from build123d import *

# Parameters (mm, degrees)
F0_W     = 25.4
F0_H     = 19.05
F0_R     = 5.08
F1_DEPTH = 2.032
F3_DEPTH = 19.05


with BuildPart() as f1:
    # F0 (on Top) → F1 (new body)
    with BuildSketch(Plane.XY):
        Rectangle(F0_W, F0_H)
        with Locations((-2.54, 0)):
            Circle(F0_R, mode=Mode.SUBTRACT)
    extrude(amount=F1_DEPTH)

    # F2 (on face) → F3 (join, through all)
    with BuildSketch(Plane.XZ.offset(9.525)):
        Polygon((10.16, 2.032), (12.7, 2.032), (12.7, 7.112), (3.482183, 7.112), (3.482183, 2.032), (4.752183, 2.032), (4.752183, 4.572), (10.16, 4.572), align=None)
    extrude(amount=-F3_DEPTH)


solid = f1.part
Design review of the part built by this model. Coordinates are the model's own, in mm. A direction names the side the tool comes from. Round coordinates to 2 decimals unless told otherwise and drop trailing zeros. Loops run counter-clockwise (first coordinate to the right, second up) from the corner with the lowest first, then second, coordinate; pieces in that order, holes last. Notation, with made-up numbers: (46.5, 30) -> (94.5, 30) arc R32 cw to (94.5, 61) -> close; hole circle Ø7 at (78, 53). An arc over 180 degrees is marked (long way). Use one line per item in the form item = value. Start each with the question number.
Q1. Draft analysis for pull direction Z (two halves, no side actions). For faces 1 (the face through (12.7, 0, 4)), 2 (the face through (8, 0, 7.112)), 3 (the face through (10.16, 0, 3)), 4 (the face through (3, 0, 0)), state which applies: +Z half, -Z half, draft (parallel to the pull), parting line (faces both ways), or undercut.
Q2. We need section B-B on x = 7.25. Give the boundary of the cut face in (y, z) (3 decimals).
Q3. We need section A-A on y = 0. Give the boundary of the cut face in (x, z).
Q4. Wall thickness on line 1 along X through (y, z) = (-0.25, 4); line 2 along Z through (x, y) = (6.25, 0.5); line 3 along Y through (x, z) = (-2.54, 1.05) (3 decimals): over which ranges is each line inside the solid? List them lowest first. Write a range as [from, to].
Q5. For pin 1 Ø8 at (x, y) = (-2, -2) entering from +Z; pin 2 Ø4 at (x, z) = (1, 5) entering from +Y; pin 3 Ø1.5 at (y, z) = (4, 3.5) entering from -X, all flat-tipped, find the tip position at first contact; note any pin that passes through.
Q6. We need section D-D on y = -7. Give the boundary of the cut face in (x, z), then the cut area to 3 significant figures.
Q7. We need section C-C on z = 3.5. Give the boundary of the cut face in (x, y) (3 decimals), then the cut area to 3 significant figures.
Q8. Machinability: for faces 5 (the face through (4.752, 0, 3)), 6 (the face through (-8, 0, 2.032)), 7 (the face through (2.305, 1.526, 1.002)), which of the approach directions +Z, -Z, +X, -X, +Y, -Y give a long, thin tool a straight path to every point of the face, cutting with its end or side? Answer none if there is none.
Calculated:
q1.face_1 = draft
q1.face_2 = +Z half
q1.face_3 = undercut
q1.face_4 = -Z half
q2.outline = (-9.525, 0) -> (9.525, 0) -> (9.525, 2.032) -> (-9.525, 2.032) -> close; (-9.525, 4.572) -> (9.525, 4.572) -> (9.525, 7.112) -> (-9.525, 7.112) -> close
q3.outline = (-12.7, 0) -> (-7.62, 0) -> (-7.62, 2.03) -> (-12.7, 2.03) -> close; (2.54, 0) -> (12.7, 0) -> (12.7, 7.11) -> (3.48, 7.11) -> (3.48, 2.03) -> (2.54, 2.03) -> close; hole (4.75, 2.03) -> (10.16, 2.03) -> (10.16, 4.57) -> (4.75, 4.57) -> close
q4.line_1 = [3.48, 4.75], [10.16, 12.7]
q4.line_2 = [0, 2.03], [4.57, 7.11]
q4.line_3 = [-9.525, -5.08], [5.08, 9.525]
q5.pin_1 = 2.03
q5.pin_2 = through
q5.pin_3 = 3.48
q6.outline = (-12.7, 0) -> (12.7, 0) -> (12.7, 7.11) -> (3.48, 7.11) -> (3.48, 2.03) -> (-12.7, 2.03) -> close; hole (4.75, 2.03) -> (10.16, 2.03) -> (10.16, 4.57) -> (4.75, 4.57) -> close
q6.area = 84.7 mm²
q7.outline = (3.482, -9.525) -> (4.752, -9.525) -> (4.752, 9.525) -> (3.482, 9.525) -> close; (10.16, -9.525) -> (12.7, -9.525) -> (12.7, 9.525) -> (10.16, 9.525) -> close
q7.area = 72.6 mm²
q8.face_5 = +Y, -Y
q8.face_6 = +Z, -X, +Y, -Y
q8.face_7 = +Z, -Z
